Source: CAD feature listing. Evaluate the final solid. Frame: model axes, mm. Give positions to 0.01 mm unless a question says otherwise; leave off trailing zeros. Write each loop counter-clockwise with the first axis right and the second up, starting at its lowest first coordinate (ties: lowest second). Pieces come first, ordered by that corner, then holes.
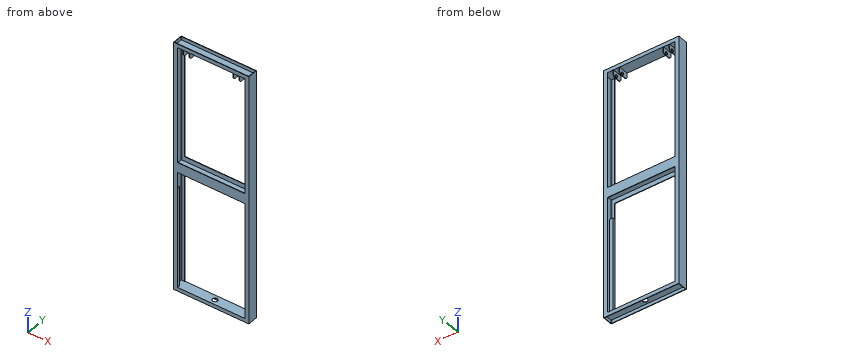
```python
from build123d import *

# Parameters (mm, degrees)
EXTRUDE_1_DEPTH          = 5000
EXTRUDE_3_DEPTH          = 1500
EXTRUDE_START            = -5000
EXTRUDE_4_DEPTH          = 5000
SKETCH_5_W               = 10
SKETCH_5_H               = 130
EXTRUDE_5_DEPTH          = 200
CUT_EXTRUDE_1_DEPTH      = 1006
CUT_EXTRUDE_1_DEPTH_BACK = 147
SKETCH_6_R               = 30
FILLET_1_R               = 60
SKETCH_7_W               = 70
SKETCH_7_H               = 2000
EXTRUDE_6_DEPTH          = 48
EXTRUDE_7_REACH          = 5224.593
SKETCH_9_R               = 50
CUT_EXTRUDE_2_DEPTH      = 219
SCALE_3_SCALE            = 0.345


with BuildPart() as part:
    # 草图1 → 凸台-拉伸1 (new body)
    with BuildSketch(Plane.XY):
        with BuildLine():
            Line((0, 40.367089679), (0, -159.632910321))
            Line((0, -159.632910321), (75, -159.632910321))
            Line((75, -159.632910321), (75, -150.632910321))
            Line((75, -150.632910321), (19, -150.632910321))
            ThreePointArc((19, -150.632910321), (11.928932188, -147.703978133), (9, -140.632910321))
            Line((9, -140.632910321), (9, 21.367089679))
            ThreePointArc((9, 21.367089679), (11.928932188, 28.43815749), (19, 31.367089679))
            Line((19, 31.367089679), (75, 31.367089679))
            Line((75, 31.367089679), (75, 40.367089679))
            Line((75, 40.367089679), (0, 40.367089679))
        make_face()
    extrude(amount=EXTRUDE_1_DEPTH)

    # 草图2 → 凸台-拉伸3 (add)
    with BuildSketch(Plane.ZY):
        Polygon((5000, 40.367089679), (4925, 40.367089679), (4925, -159.632910321), (5000, -159.632910321), (5000, -150.632910321), (4934, -150.632910321), (4934, 31.367089679), (5000, 31.367089679), align=None)
        Polygon((0, -150.632910321), (0, -159.632910321), (75, -159.632910321), (75, 40.367089679), (0, 40.367089679), (0, 31.367089679), (66, 31.367089679), (66, -150.632910321), align=None)
    extrude(amount=-EXTRUDE_3_DEPTH)

    # 草图3 → 凸台-拉伸4 (add)
    with BuildSketch(Plane(origin=(0, 0, 0), x_dir=(-1, 0, 0), z_dir=(0, 0, -1)).offset(EXTRUDE_START)):
        with BuildLine():
            Line((-1500, 40.367089679), (-1425, 40.367089679))
            Line((-1425, 40.367089679), (-1425, 31.367089679))
            Line((-1425, 31.367089679), (-1481, 31.367089679))
            ThreePointArc((-1481, 31.367089679), (-1488.071067812, 28.43815749), (-1491, 21.367089679))
            Line((-1491, 21.367089679), (-1491, -140.632910321))
            ThreePointArc((-1491, -140.632910321), (-1488.071067812, -147.703978133), (-1481, -150.632910321))
            Line((-1481, -150.632910321), (-1425, -150.632910321))
            Line((-1425, -150.632910321), (-1425, -159.632910321))
            Line((-1425, -159.632910321), (-1500, -159.632910321))
            Line((-1500, -159.632910321), (-1500, 40.367089679))
        make_face()
    extrude(amount=EXTRUDE_4_DEPTH)

    # 草图5 → 凸台-拉伸5 (add)
    with BuildSketch(Plane(origin=(0, 40.367089679, 0), x_dir=(1, 0, 0), z_dir=(0, 1, 0))):
        with Locations((191, -4860)):
            Rectangle(SKETCH_5_W, SKETCH_5_H)
        with Locations((313, -4860)):
            Rectangle(SKETCH_5_W, SKETCH_5_H)
        with Locations((1309, -4860)):
            Rectangle(SKETCH_5_W, SKETCH_5_H)
        with Locations((1187, -4860)):
            Rectangle(SKETCH_5_W, SKETCH_5_H)
    extrude(amount=-EXTRUDE_5_DEPTH)

    # 草图6 → 切除-拉伸1 (cut, two sides: drawn at the far end of the back side and taken through both)
    with BuildSketch(Plane(origin=(318, 0, 0), x_dir=(0, 0, -1), z_dir=(1, 0, 0)).offset(-CUT_EXTRUDE_1_DEPTH_BACK)):
        with Locations((-4845, -39.632910321)):
            Circle(SKETCH_6_R)
    extrude(amount=CUT_EXTRUDE_1_DEPTH + CUT_EXTRUDE_1_DEPTH_BACK, mode=Mode.SUBTRACT)

    # 圆角1
    fillet_1_edges = [part.edges().sort_by_distance(p)[0] for p in [
        (191, -159.632910321, 4795),
        (191, 40.367089679, 4795),
        (313, -159.632910321, 4795),
        (313, 40.367089679, 4795),
        (1187, -159.632910321, 4795),
        (1187, 40.367089679, 4795),
        (1309, -159.632910321, 4795),
        (1309, 40.367089679, 4795),
    ]]
    fillet(fillet_1_edges, radius=FILLET_1_R)

    # 草图7 → 凸台-拉伸6 (add)
    with BuildSketch(Plane(origin=(0, -150.632910321, 0), x_dir=(1, 0, 0), z_dir=(0, 1, 0))):
        with Locations((40, -1075)):
            Rectangle(SKETCH_7_W, SKETCH_7_H)
        with Locations((1460, -1075)):
            Rectangle(SKETCH_7_W, SKETCH_7_H)
    extrude(amount=EXTRUDE_6_DEPTH)

    # 凸台-拉伸7: up to this face of the body (flat: up to its plane)
    extrude_7_end = Plane(part.part.faces().sort_by_distance((1491, -52.993485212, 2652.59969001))[0])
    # 草图8 → 凸台-拉伸7 (add, up to the picked face)
    with BuildSketch(Plane.ZY, mode=Mode.PRIVATE) as extrude_7_sk1:
        Polygon((2400, 40.367089679), (2600, 40.367089679), (2600, 31.367089679), (2509, 31.367089679), (2509, -150.632910321), (2600, -150.632910321), (2600, -159.632910321), (2400, -159.632910321), (2400, -150.632910321), (2491, -150.632910321), (2491, 31.367089679), (2400, 31.367089679), align=None)
    extrude_7_tool1 = split(extrude(extrude_7_sk1.sketch, amount=-EXTRUDE_7_REACH, mode=Mode.PRIVATE), bisect_by=extrude_7_end, keep=Keep.BOTH, mode=Mode.PRIVATE)
    add(extrude_7_tool1.solids().sort_by(Axis((0, -59.63291, 2500), (1, 0, 0)))[0])

    # 草图9 → 切除-拉伸2 (cut)
    with BuildSketch(Plane(origin=(0, 0, 66), x_dir=(-1, 0, 0), z_dir=(0, 0, -1))):
        with Locations((-750, -59.632910321)):
            Circle(SKETCH_9_R)
    extrude(amount=-CUT_EXTRUDE_2_DEPTH, mode=Mode.SUBTRACT)


with BuildPart() as part_1:
    # 缩放比例3: scaled about (0, 0, 0)
    add(part.part.scale(SCALE_3_SCALE))


solid = part_1.part
```
1. Section query A-A (z = 239.5). Return loops of the section in (x, y) (3 decimals).
2. Section query D-D (z = 1398). Return loops of the section in (x, y) (3 decimals), plus the area to 3 significant figures.
3. Section query B-B (x = 258.75). Give the number of separate pieces and of enclosed holes in the cut face, plus the area to 3 significant figures.
4. Pin query (flat end, axial travel): P1, Ø8, axis at x = 102, y = -27, coming from the +Z side; P2, Ø1, axis at x = 409.5, y = -17.5, coming from the -Z side. Return the tip coordinate at first contact, or that it passes through.
5. Line query: probe 1 along Z at (x, y) = (431, 5.5) (3 decimals); probe 2 along X at (y, z) = (-43, 918) (3 decimals); probe 3 along Y at (x, z) = (258.75, 23.85). Output: solid intervals per line, ascending.
6. Section query C-C (x = 140). Return loops of the section in (y, z) (3 decimals).
The answers:
1. outline: (0, -55.073) - (25.875, -55.073) - (25.875, -35.408) - (3.105, -35.408) - (3.105, 7.372) arc R3.45 cw to (6.555, 10.822) - (25.875, 10.822) - (25.875, 13.927) - (0, 13.927) - close; (491.625, -55.073) - (517.5, -55.073) - (517.5, 13.927) - (491.625, 13.927) - (491.625, 10.822) - (510.945, 10.822) arc R3.45 cw to (514.395, 7.372) - (514.395, -35.408) - (491.625, -35.408) - close
2. outline: (0, -55.073) - (25.875, -55.073) - (25.875, -51.968) - (6.555, -51.968) arc R3.45 cw to (3.105, -48.518) - (3.105, 7.372) arc R3.45 cw to (6.555, 10.822) - (25.875, 10.822) - (25.875, 13.927) - (0, 13.927) - close; (491.625, -55.073) - (517.5, -55.073) - (517.5, 13.927) - (491.625, 13.927) - (491.625, 10.822) - (510.945, 10.822) arc R3.45 cw to (514.395, 7.372) - (514.395, -48.518) arc R3.45 cw to (510.945, -51.968) - (491.625, -51.968) - close
2. area: 722 mm2
3. separate pieces: 4
3. enclosed holes: 0
3. area: 1,420 mm2
4. P1: stops at z = 1702.23
4. P2: stops at z = 22.77
5. probe 1: z = 22.77 to 25.875, 859.395 to 865.605, 1699.125 to 1702.23
5. probe 2: x = 0 to 3.105, 514.395 to 517.5
5. probe 3: y = -55.07 to -37.82, -3.32 to 13.93
6. outline: (-55.073, 0) - (-51.968, 0) - (-51.968, 22.77) - (10.822, 22.77) - (10.822, 0) - (13.927, 0) - (13.927, 25.875) - (-55.073, 25.875) - close; (-55.073, 828) - (-51.968, 828) - (-51.968, 859.395) - (10.822, 859.395) - (10.822, 828) - (13.927, 828) - (13.927, 897) - (10.822, 897) - (10.822, 865.605) - (-51.968, 865.605) - (-51.968, 897) - (-55.073, 897) - close; (-55.073, 1699.125) - (13.927, 1699.125) - (13.927, 1725) - (10.822, 1725) - (10.822, 1702.23) - (-51.968, 1702.23) - (-51.968, 1725) - (-55.073, 1725) - close
